from build123d import *

# Parameters (mm, degrees)
BOSS_EXTRUDE1_DEPTH = 10
SKETCH2_R           = 4
CUT_EXTRUDE1_DEPTH  = 5
SKETCH3_R           = 2.5
CUT_EXTRUDE2_DEPTH  = 6
SKETCH5_R           = 4
CUT_EXTRUDE3_DEPTH  = 5
SKETCH6_R           = 2.5
CUT_EXTRUDE4_DEPTH  = 5


with BuildPart() as part:
    # Sketch1 → Boss-Extrude1 (new body)
    with BuildSketch(Plane(origin=(0, 0, 0), x_dir=(1, 0, 0), z_dir=(0, 1, 0))):
        Polygon((0, 0), (38, 0), (38, 20), (58, 20), (58, 165), (-20, 165), (-20, 20), (0, 20), align=None)
    extrude(amount=BOSS_EXTRUDE1_DEPTH)

    # Sketch2 → Cut-Extrude1 (cut)
    with BuildSketch(Plane(origin=(0, 10, 0), x_dir=(1, 0, 0), z_dir=(0, 1, 0))):
        with Locations((9, 16.329867595)):
            Circle(SKETCH2_R)
        with Locations((29, 16.329867595)):
            Circle(SKETCH2_R)
    extrude(amount=-CUT_EXTRUDE1_DEPTH, mode=Mode.SUBTRACT)

    # Sketch3 → Cut-Extrude2 (cut, through all)
    with BuildSketch(Plane(origin=(0, 5, 0), x_dir=(1, 0, 0), z_dir=(0, 1, 0))):
        with Locations((9, 16.329867595)):
            Circle(SKETCH3_R)
        with Locations((29, 16.329867595)):
            Circle(SKETCH3_R)
    extrude(amount=-CUT_EXTRUDE2_DEPTH, mode=Mode.SUBTRACT)

    # Sketch5 → Cut-Extrude3 (cut)
    with BuildSketch(Plane.XZ):
        with Locations((-15, -131)):
            Circle(SKETCH5_R)
        with Locations((53, -131)):
            Circle(SKETCH5_R)
        with Locations((-12, -28)):
            Circle(SKETCH5_R)
        with Locations((50, -28)):
            Circle(SKETCH5_R)
        with Locations((-12, -62)):
            Circle(SKETCH5_R)
        with Locations((50, -62)):
            Circle(SKETCH5_R)
    extrude(amount=-CUT_EXTRUDE3_DEPTH, mode=Mode.SUBTRACT)

    # Sketch6 → Cut-Extrude4 (cut)
    with BuildSketch(Plane.XZ.offset(-5)):
        with Locations((-15, -131)):
            Circle(SKETCH6_R)
        with Locations((53, -131)):
            Circle(SKETCH6_R)
        with Locations((-12, -28)):
            Circle(SKETCH6_R)
        with Locations((50, -28)):
            Circle(SKETCH6_R)
        with Locations((-12, -62)):
            Circle(SKETCH6_R)
        with Locations((50, -62)):
            Circle(SKETCH6_R)
    extrude(amount=-CUT_EXTRUDE4_DEPTH, mode=Mode.SUBTRACT)


solid = part.part
Input: part model. Units: mm. Frame: model coordinates. A direction names the side the tool comes from. Coordinates: 2 decimals unless noted, no trailing zeros. Loops run counter-clockwise (first coordinate to the right, second up) from the corner with the lowest first, then second, coordinate; pieces in that order, holes last. Notation, with made-up numbers: (32, 30) -> (84, 30) arc R30 cw to (84, 55) -> close; hole circle Ø11 at (75.5, 5.25). An arc over 180 degrees is marked (long way). Write item = value, one per line. Start each with the question number.
Item 1: Material intervals for line 1 (X direction, y = 6.1, z = -131); line 2 (Z direction, x = 50, y = 3.75); line 3 (Z direction, x = 53, y = 1.85), sorted ascending.
Item 2: Reachability of faces 5 (the face through (49.133, 2.465, -65.905)), 6 (the face through (-12.33, 7.46, -25.52)), 7 (the face through (0, 5, -10)), 8 (the face through (32, 5, -16)), 9 (the face through (58, 5, -91)) from +Z, -Z, +X, -X, +Y, -Y: full face, straight path, thin tool, end or side. Return the list, or none.
Item 3: Cut plane C-C, the plane y = 1.75. Count the separate pieces of the cut face and the enclosed holes in it, plus the area to 3 significant figures.
Item 4: Cut plane A-A, the plane x = 29. Return loops of the section in (y, z).
Item 5: Cut plane B-B, the plane z = -28. Return loops of the section in (x, y).
Item 6: Mould query, pull axis Z, two halves, no side actions, for faces 1 (the face through (-14.5, 7.5, -61.9)), 2 (the face through (51.34, 7.46, -25.89)), 3 (the face through (-10, 5, -20)), 4 (the face through (38, 5, -10)). Classes: pulls with the +Z half, pulls with the -Z half, needs draft (parallel to the pull), parting line crosses it, or undercut.
Item 7: First-contact query: P1, Ø2.5, axis at x = 54.5, z = -131.5, coming from the -Y side; P2, Ø6.5, axis at x = 9, z = -16.33, coming from the +Y side; P3, Ø5, axis at x = 46, y = 2.5, coming from the +Z side. Flat tips, straight axial feed; report the tip coordinate or a pass-through.
Ans:
q1.line_1 = -20 to -17.5, -12.5 to 50.5, 55.5 to 58
q1.line_2 = -165 to -133.65, -128.35 to -66, -58 to -32, -24 to -20
q1.line_3 = -165 to -135, -127 to -64.65, -59.35 to -30.65, -25.35 to -20
q2.face_5 = -Y
q2.face_6 = +Y, -Y
q2.face_7 = +Z, -X, +Y, -Y
q2.face_8 = +Y
q2.face_9 = +Z, -Z, +X, +Y, -Y
q3.separate_pieces = 1
q3.enclosed_holes = 8
q3.area = 11,700 mm²
q4.outline = (0, -165) -> (10, -165) -> (10, -20.33) -> (5, -20.33) -> (5, -18.83) -> (0, -18.83) -> close; (0, -13.83) -> (5, -13.83) -> (5, -12.33) -> (10, -12.33) -> (10, 0) -> (0, 0) -> close
q5.outline = (-20, 0) -> (-16, 0) -> (-16, 5) -> (-14.5, 5) -> (-14.5, 10) -> (-20, 10) -> close; (-9.5, 5) -> (-8, 5) -> (-8, 0) -> (46, 0) -> (46, 5) -> (47.5, 5) -> (47.5, 10) -> (-9.5, 10) -> close; (52.5, 5) -> (54, 5) -> (54, 0) -> (58, 0) -> (58, 10) -> (52.5, 10) -> close
q6.face_1 = undercut
q6.face_2 = undercut
q6.face_3 = pulls with the +Z half
q6.face_4 = needs draft
q7.P1 = 5
q7.P2 = 5
q7.P3 = -20
